The listing builds one solid part. Answer for the finished solid, in the listing's coordinates (mm). Give positions to 0.01 mm unless a question says otherwise; leave off trailing zeros. Loops run counter-clockwise (first coordinate to the right, second up) from the corner with the lowest first, then second, coordinate; pieces in that order, holes last. Notation, with made-up numbers: (38, -7) - (44, -7) arc R10 cw to (44, 12) - close; hole circle Ø1 at (-30.5, 83.5). An arc over 180 degrees is marked (long way). Write each question's results on one line, items separated by ' | '.
from build123d import *

# Parameters (mm, degrees)
F0_W     = 1.66
F0_H     = 1.1787281516
F0_W_2   = 1.5189777559
F0_H_2   = 1.66
F1_DEPTH = 71.45
F2_R     = 0.15
F3_R     = 0.15


with BuildPart() as f1:
    # F0 (on Top) → F1 (new body)
    with BuildSketch(Plane.XY):
        with Locations((0, 1.4193640758)):
            Rectangle(F0_W, F0_H)
        with Locations((1.5894888779, 0)):
            Rectangle(F0_W_2, F0_H_2)
        Rectangle(F0_W, F0_H_2)
        with Locations((-1.5894888779, 0)):
            Rectangle(F0_W_2, F0_H_2)
        with Locations((0, -1.4193640758)):
            Rectangle(F0_W, F0_H)
    extrude(amount=F1_DEPTH)

    # F2
    f2_edges = [f1.edges().sort_by_distance(p)[0] for p in [
        (-2.348978, 0, 71.45),
        (-1.589489, 0.83, 71.45),
        (-0.83, 1.419364, 71.45),
        (0, 2.008728, 71.45),
        (0.83, 1.419364, 71.45),
        (2.348978, 0, 71.45),
        (1.589489, 0.83, 71.45),
        (1.589489, -0.83, 71.45),
        (0.83, -1.419364, 71.45),
        (0, -2.008728, 71.45),
        (-0.83, -1.419364, 71.45),
        (-1.589489, -0.83, 71.45),
    ]]
    fillet(f2_edges, radius=F2_R)

    # F3
    f3_edges = [f1.edges().sort_by_distance(p)[0] for p in [
        (-1.589489, -0.83, 0),
        (-2.348978, 0, 0),
        (-1.589489, 0.83, 0),
        (-0.83, 1.419364, 0),
        (0, 2.008728, 0),
        (0.83, 1.419364, 0),
        (1.589489, 0.83, 0),
        (2.348978, 0, 0),
        (1.589489, -0.83, 0),
        (0.83, -1.419364, 0),
        (0, -2.008728, 0),
        (-0.83, -1.419364, 0),
    ]]
    fillet(f3_edges, radius=F3_R)


solid = f1.part
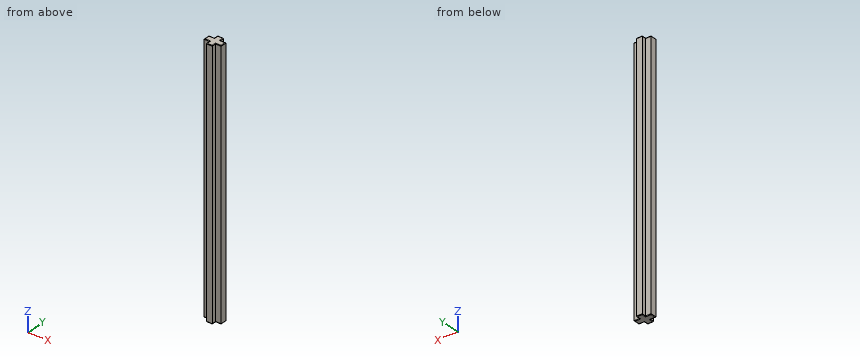
Item 1: A cutting plane is placed at B-B, the plane z = 40.5. Determine the outline of the cut face in (x, y), plus the area to 3 significant figures.
Values found:
outline: (-2.35, -0.83) - (-0.83, -0.83) - (-0.83, -2.01) - (0.83, -2.01) - (0.83, -0.83) - (2.35, -0.83) - (2.35, 0.83) - (0.83, 0.83) - (0.83, 2.01) - (-0.83, 2.01) - (-0.83, 0.83) - (-2.35, 0.83) - close | area: 11.7 mm²
Item 2: Flat-ended cylindrical pins translate along their axes: P1, Ø0.8, axis at x = 1.5, z = 33, coming from the +Y side; P2, Ø0.6, axis at y = -1.5, z = 29.5, coming from the -X side; P3, Ø0.5, axis at x = -1.5, z = 21.5, coming from the -Y side. Find the tip coordinate at first contact, or state that the pin passes through.
Values found:
P1: stops at y = 0.83 | P2: stops at x = -0.83 | P3: stops at y = -0.83
Item 3: Find the intervals of material crossed by line 1 along X through (y, z) = (0.9, 29.5); line 2 along Z through (x, y) = (1.6, -0.75), in increasing order. Write a range as [from, to].
Values found:
line 1: x = [-0.83, 0.83] | line 2: z = [0.02, 71.43]
Item 4: A cutting plane is placed at A-A, the plane x = 1.6. Determine the outline of the cut face in (y, z).
Values found:
outline: (-0.83, 0.15) arc R0.15 ccw to (-0.68, 0) - (0.68, 0) arc R0.15 ccw to (0.83, 0.15) - (0.83, 71.3) arc R0.15 ccw to (0.68, 71.45) - (-0.68, 71.45) arc R0.15 ccw to (-0.83, 71.3) - close
